The figure shows three views and two pictorial views of one solid part (mm, origin at its lowest corner). Answer the questions. Give positions to 0.01 mm unless a question says otherwise; leave off trailing zeros. Order: outer loops, then holes, each group sorted by start corner. A loop starts at its lowest first (then second) coordinate and runs counter-clockwise, first axis right, second up. Notation, with made-up numbers: (75.25, -34.5) - (134.25, -34.5) arc R9 cw to (134.25, -26.5) - close; hole circle Ø6 at (84.5, 82). An arc over 180 degrees is marked (long way). Use a Markdown table: item, result. Add a question column.
1. Consider L1, parallel to Y at x = 7.75, z = 1.75; L2, parallel to X at y = 3.5, z = 0.9; L3, parallel to Y at x = 3.5, z = 2.5. Determine where each line is inside the solid, lowest interval first.
2. Flat-ended cylindrical pins translate along their axes: P1, Ø0.5, axis at x = 11, y = 1.5, coming from the +Z side; P2, Ø1.5, axis at x = 3.5, y = 3.5, coming from the +Z side; P3, Ø1.1, axis at x = 11, y = 5.5, coming from the +Z side. Find the tip coordinate at first contact, or state that the pin passes through.
3. A cutting plane is placed at A-A on y = 4.5. Determine the outline of the cut face in (x, z) (3 decimals).
4. For a pull along Y with two mould halves and no side action, classify the marked faces 1, 2, 3 and 4 as released by +Y, released by -Y, zero draft, split by the parting line, or undercut.
5. A cutting plane is placed at D-D on y = 7.75. Determine the outline of the cut face in (x, z).
6. A cutting plane is placed at B-B on x = 1.75. Determine the outline of the cut face in (y, z).
7. A cutting plane is placed at C-C on z = 0.65. Determine the outline of the cut face in (x, y) (3 decimals), and give its area (3 significant figures).
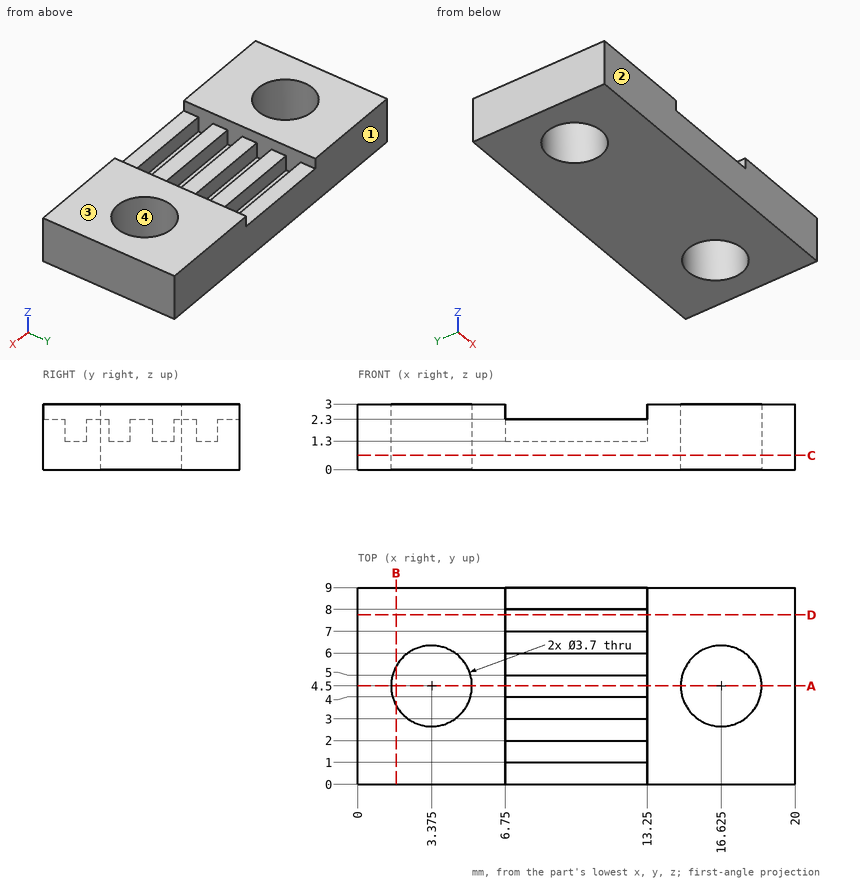
Output values:
| question | item | result |
|---|---|---|
| 1 | L1 | 0 to 1, 2 to 3, 4 to 5, 6 to 7, 8 to 9 |
| 1 | L2 | 0 to 1.82, 4.93 to 15.07, 18.18 to 20 |
| 1 | L3 | 0 to 2.65, 6.35 to 9 |
| 2 | P1 | z = 1.3 |
| 2 | P2 | through |
| 2 | P3 | z = 2.3 |
| 3 | outline | (0, 0) - (1.525, 0) - (1.525, 3) - (0, 3) - close; (5.225, 0) - (14.775, 0) - (14.775, 3) - (13.25, 3) - (13.25, 2.3) - (6.75, 2.3) - (6.75, 3) - (5.225, 3) - close; (18.475, 0) - (20, 0) - (20, 3) - (18.475, 3) - close |
| 4 | face 1 | released by +Y |
| 4 | face 2 | released by -Y |
| 4 | face 3 | zero draft |
| 4 | face 4 | undercut |
| 5 | outline | (0, 0) - (20, 0) - (20, 3) - (13.25, 3) - (13.25, 1.3) - (6.75, 1.3) - (6.75, 3) - (0, 3) - close |
| 6 | outline | (0, 0) - (3.62, 0) - (3.62, 3) - (0, 3) - close; (5.38, 0) - (9, 0) - (9, 3) - (5.38, 3) - close |
| 7 | outline | (0, 0) - (20, 0) - (20, 9) - (0, 9) - close; hole circle Ø3.7 at (3.375, 4.5); hole circle Ø3.7 at (16.625, 4.5) |
| 7 | area | 158 mm² |
